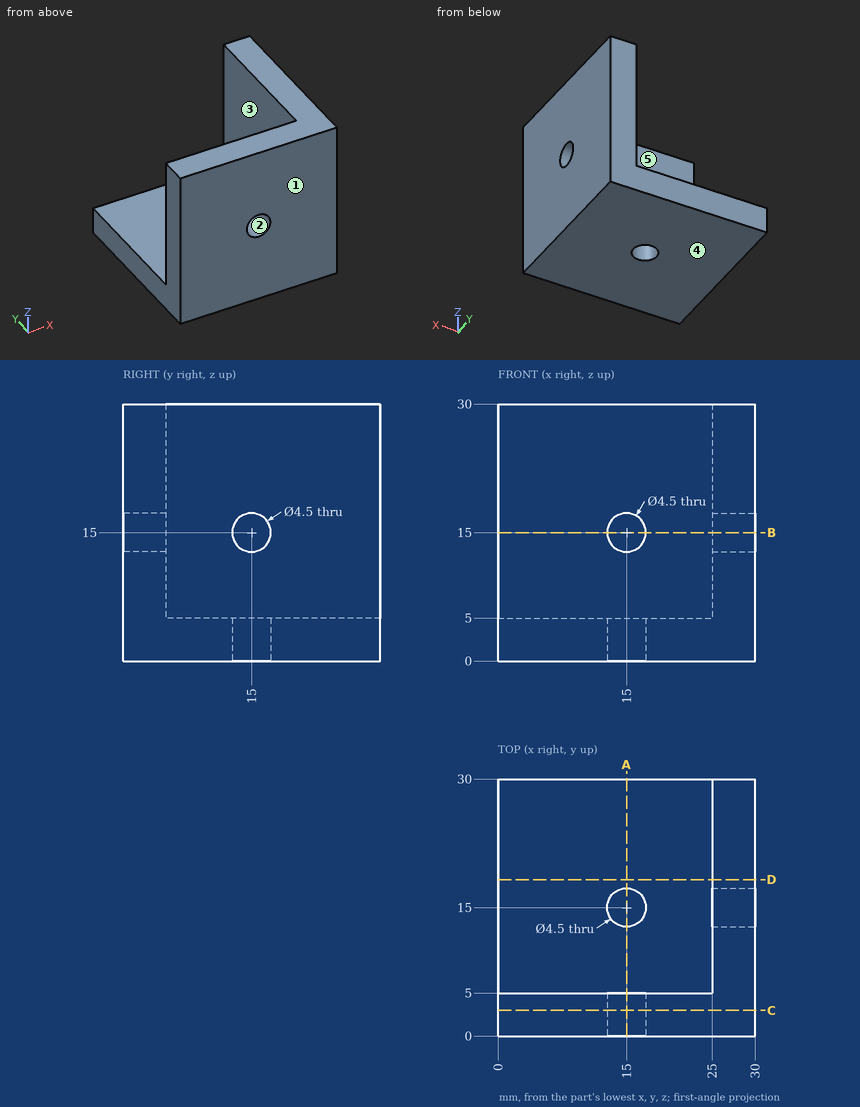
Study the drawing (mm; zero at the part's minimum x, y, z) and answer. A direction names the side the tool comes from. Give positions to 0.01 mm unless a question says otherwise; leave off trailing zeros. Order: outer loops, then holes, each group sorted by start corner. A loop starts at its lowest first (then second) coordinate and runs counter-clockwise, first axis right, second up. Notation, with made-up numbers: (83, 48) - (121, 48) arc R28 cw to (121, 83) - close; hole circle Ø3 at (-26.5, 32.25). An arc over 180 degrees is marked (long way). Answer in a Markdown table with one row per item. Add a question column.
Q1. The part is cut by section B-B (z = 15). Determine the outline of the cut face in (x, y).
Q2. For a pull along X with two mould halves and no side action, classify the marked faces 1, 2 and 3 as released by +X, released by -X, zero draft, split by the parting line, or undercut.
Q3. The part is cut by section C-C (y = 3). Determine the outline of the cut face in (x, z).
Q4. The part is cut by section A-A (x = 15). Determine the outline of the cut face in (y, z).
Q5. Find the intervals of material crossed by line 1 along Z through (x, y) = (26.45, 15), in increasing order. Write a range as [from, to].
Q6. Given P1, Ø7.5, axis at x = 12, y = 19, coming from the +Z side; P2, Ø7.5, axis at y = 23, z = 17.5, coming from the -X side; P3, Ø1.5, axis at x = 4, z = 7, coming from the +Y side, each flat-ended and moving along its own axis, determine where each tip first touches the part or whether it passes through.
Q7. Which of the six approach directions +Z, -Z, +X, -X, +Y, -Y give full straight-line access (tool end or side, diameter ignored) to the marked faces 4 and 5?
Q8. The part is cut by section D-D (y = 18.25). Determine the outline of the cut face in (x, z).
Determined:
| question | item | result |
|---|---|---|
| 1 | outline | (0, 0) - (12.75, 0) - (12.75, 5) - (0, 5) - close; (17.25, 0) - (30, 0) - (30, 12.75) - (25, 12.75) - (25, 5) - (17.25, 5) - close; (25, 17.25) - (30, 17.25) - (30, 30) - (25, 30) - close |
| 2 | face 1 | zero draft |
| 2 | face 2 | undercut |
| 2 | face 3 | released by -X |
| 3 | outline | (0, 0) - (30, 0) - (30, 30) - (0, 30) - close; hole circle Ø4.5 at (15, 15) |
| 4 | outline | (0, 0) - (12.75, 0) - (12.75, 5) - (5, 5) - (5, 12.75) - (0, 12.75) - close; (0, 17.25) - (5, 17.25) - (5, 30) - (0, 30) - close; (17.25, 0) - (30, 0) - (30, 5) - (17.25, 5) - close |
| 5 | line 1 | z = [0, 12.75], [17.25, 30] |
| 6 | P1 | stops at z = 5 |
| 6 | P2 | stops at x = 25 |
| 6 | P3 | stops at y = 5 |
| 7 | face 4 | -Z, +X, -X, +Y, -Y |
| 7 | face 5 | +Z, -X, +Y |
| 8 | outline | (0, 0) - (30, 0) - (30, 30) - (25, 30) - (25, 5) - (0, 5) - close |
